The model under review builds one solid part; all positions refer to its coordinate system, in mm. Face numbers are marked on the shaded views. Round coordinates to 2 decimals unless told otherwise and drop trailing zeros. Order: outer loops, then holes, each group sorted by start corner. A loop starts at its lowest first (then second) coordinate and runs counter-clockwise, first axis right, second up. Notation, with made-up numbers: M 88.5,23 L 112.5,23 A7 cw 112.5,27 Z; hole C -24,-6.5 d4. An arc over 180 degrees is marked long. One line per item, written item: value. Start each with the question number.
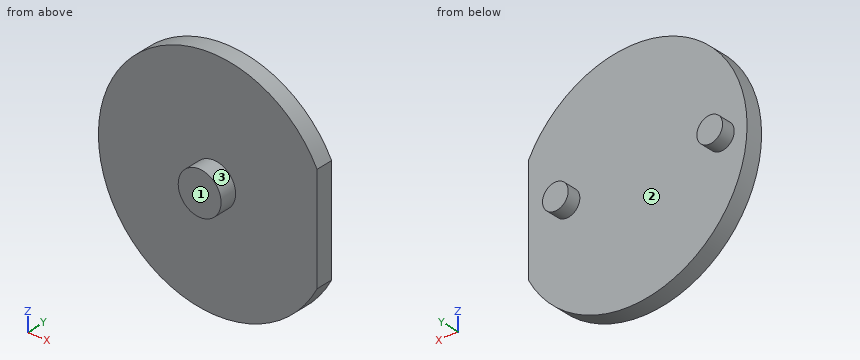
from build123d import *

# Parameters (mm, degrees)
SALIENTE_EXTRUIR1_DEPTH = 2
CROQUIS3_R              = 1.5
SALIENTE_EXTRUIR2_DEPTH = 1.6
CROQUIS4_R              = 2.5
SALIENTE_EXTRUIR3_DEPTH = 2


with BuildPart() as part:
    # Croquis2 → Saliente-Extruir1 (new body)
    with BuildSketch(Plane(origin=(0, 0, 0), x_dir=(1, 0, 0), z_dir=(0, 1, 0))):
        with BuildLine():
            Line((12, 6.184658438), (12, -6.184658438))
            ThreePointArc((12, -6.184658438), (-13.5, 0), (12, 6.184658438))
        make_face()
    extrude(amount=SALIENTE_EXTRUIR1_DEPTH)

    # Croquis3 → Saliente-Extruir2 (add)
    with BuildSketch(Plane(origin=(0, 2, 0), x_dir=(1, 0, 0), z_dir=(0, 1, 0))):
        with Locations(Location((-10.5, 0, 0), (0, 0, 270))):
            Circle(CROQUIS3_R)
        with Locations(Location((7.5, 0, 0), (0, 0, 270))):
            Circle(CROQUIS3_R)
    extrude(amount=SALIENTE_EXTRUIR2_DEPTH)

    # Croquis4 → Saliente-Extruir3 (add)
    with BuildSketch(Plane.XZ):
        with Locations(Location((0, 0, 0), (0, 0, 270))):
            Circle(CROQUIS4_R)
    extrude(amount=SALIENTE_EXTRUIR3_DEPTH)


solid = part.part
Item 1: Consider section B-B, the plane z = 0. Give the boundary of the cut face in (x, y), then the cut area to 3 significant figures.
Item 2: Wall thickness on L1, parallel to Y at x = -8.75, z = -3.75; L2, parallel to X at y = 2.5, z = -1; L3, parallel to Z at x = 7.75, y = 2.6: over which ranges is each line inside the solid? List them lowest first.
Item 3: The part is to be moulded in two halves that separate along Y. For the marked faces 1, 2 and 3, say which applies: pulls with the +Y half, pulls with the -Y half, needs draft (parallel to the pull), parting line crosses it, or undercut.
Item 4: Consider section C-C, the plane y = 1.35. Give the boundary of the cut face in (x, z), then the cut area to 3 significant figures.
Item 5: Clearance check with flat-ended pins moving along their axes: P1, Ø1, axis at y = 3, z = 9.5, coming from the -X side; P2, Ø1.5, axis at y = 3, z = 1.5, coming from the -X side; P3, Ø1, axis at y = 1.5, z = -7, coming from the +X side; P4, Ø1.5, axis at y = 2, z = -8, coming from the -X side. State where each tip first meets the part, or that it passes through.
Item 6: Consider section D-D, the plane x = -11.25. Give the boundary of the cut face in (y, z).
Item 7: Consider section A-A, the plane x = 0. Give the boundary of the cut face in (y, z), then the cut area to 3 significant figures.
Computed:
1. outline: M -13.5,0 L -2.5,0 L -2.5,-2 L 2.5,-2 L 2.5,0 L 12,0 L 12,2 L 9,2 L 9,3.6 L 6,3.6 L 6,2 L -9,2 L -9,3.6 L -12,3.6 L -12,2 L -13.5,2 Z
1. area: 70.6 mm^2
2. L1: y = 0 to 2
2. L2: x = -11.62 to -9.38, 6.38 to 8.62
2. L3: z = -1.48 to 1.48
3. face 1: pulls with the -Y half
3. face 2: pulls with the +Y half
3. face 3: needs draft
4. outline: M 12,-6.18 L 12,6.18 A13.5 ccw long Z
4. area: 560 mm^2
5. P1: passes through
5. P2: stops at x = -11.8
5. P3: stops at x = 11.83
5. P4: stops at x = -11.39
6. outline: M 0,-7.46 L 2,-7.46 L 2,-1.3 L 3.6,-1.3 L 3.6,1.3 L 2,1.3 L 2,7.46 L 0,7.46 Z
7. outline: M -2,-2.5 L 0,-2.5 L 0,-13.5 L 2,-13.5 L 2,13.5 L 0,13.5 L 0,2.5 L -2,2.5 Z
7. area: 64.0 mm^2
